```python
from build123d import *

# Parameters (mm, degrees)
F0_R     = 6.35
F1_DEPTH = 31.75
F2_R     = 7.9375
F3_DEPTH = 9.525
F4_DEPTH = 9.525


with BuildPart() as f1:
    # F0 (on Front) → F1 (new body)
    with BuildSketch(Plane.XZ):
        with BuildLine():
            ThreePointArc((-45.625926, 31.75), (-61.553538, 17.067408), (-48.212963, 0))
            Line((-48.212963, 0), (52.916662, 0))
            Line((52.916662, 0), (52.916662, 9.525))
            Line((52.916662, 9.525), (34.337035, 9.525))
            Line((34.337035, 9.525), (34.337035, 22.225))
            Line((34.337035, 22.225), (52.681481, 22.225))
            Line((52.681481, 22.225), (52.681481, 31.75))
            Line((52.681481, 31.75), (-45.625926, 31.75))
        make_face()
        with Locations((-45.625926, 15.769602)):
            Circle(F0_R, mode=Mode.SUBTRACT)
    extrude(amount=-F1_DEPTH)

    # F2 (on Top) → F3 (join, through all)
    with BuildSketch(Plane.XY):
        with BuildLine():
            ThreePointArc((52.916662, 31.75), (37.041662, 15.875), (52.916662, 0))
            ThreePointArc((52.916662, 0), (64.141982, 4.64968), (68.791662, 15.875))
            ThreePointArc((68.791662, 15.875), (64.141982, 27.10032), (52.916662, 31.75))
        make_face()
        with Locations((52.916662, 15.875)):
            Circle(F2_R, mode=Mode.SUBTRACT)
    extrude(amount=F3_DEPTH)

    # F2 (on Top) → F4 (cut, through all)
    with BuildSketch(Plane.XY):
        with Locations((52.916662, 15.875)):
            Circle(F2_R)
    extrude(amount=F4_DEPTH, mode=Mode.SUBTRACT)


solid = f1.part
```
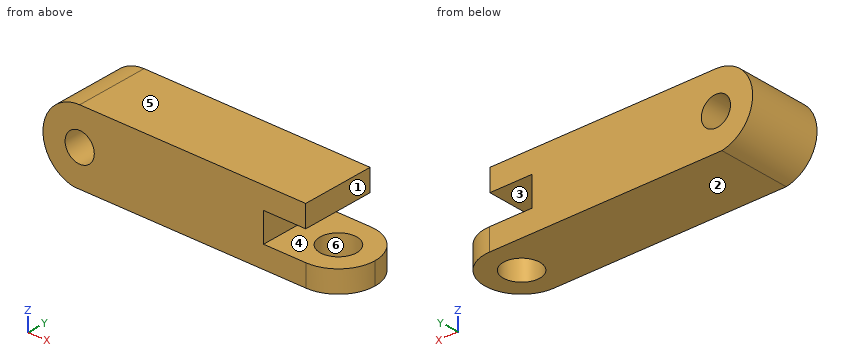
Could you check a few things on this model? Use its own coordinates, in mm. Face numbers are marked on the shaded views. A direction names the side the tool comes from. Round coordinates to 2 decimals unless told otherwise and drop trailing zeros. Loops run counter-clockwise (first coordinate to the right, second up) from the corner with the lowest first, then second, coordinate; pieces in that order, holes last.
Q1. I want a section at B-B (y = 14.5). Write out the boundary of the cut face in (x, z) (3 decimals), and give its area (3 significant figures).
Q2. For P1, Ø5, axis at x = 48.5, z = 11, coming from the +Y side; P2, Ø3, axis at y = 9, z = 26.5, coming from the +X side; P3, Ø5, axis at y = 4, z = 12, coming from the -X side; P4, Ø12, axis at y = 22.5, z = 8, coming from the -X side, each with a flat end and sliding along its axis, tell me the tip position at first contact or that it passes through.
Q3. I want a section at D-D (y = 4). Write out the boundary of the cut face in (x, z) (3 decimals).
Q4. On a 3-axis mill with a long thin cutter (end or side, diameter ignored), from which of +Z, -Z, +X, -X, +Y, -Y can I reach the whole of each face in a straight line? I mean the marked faces 4, 5 and 6. Say none if no direction works.
Q5. Please list where these lines run through material, in increasing order: L1, parallel to X at y = 27, z = 16; L2, parallel to Z at x = 38, y = 21.5 (3 decimals); L3, parallel to X at y = 19, z = 3.5.
Q6. I want a section at C-C (z = 20). Write out the boundary of the cut face in (x, y), and give its area (3 significant figures).
Q7. Thinking about a two-plate mould opening in Z: for the marked faces 1, 2 and 3, which applies, pulls with the +Z half, pulls with the -Z half, needs draft (parallel to the pull), parting line crosses it, or undercut?
Q8. I want a section at A-A (x = 42.5). Write out the boundary of the cut face in (y, z) (3 decimals), and give its area (3 significant figures).
Answer below:
1. outline: (-48.213, 0) - (45.099, 0) - (45.099, 9.525) - (34.337, 9.525) - (34.337, 22.225) - (52.681, 22.225) - (52.681, 31.75) - (-45.626, 31.75) arc R15.98 ccw to start; (60.734, 0) - (68.732, 0) - (68.732, 9.525) - (60.734, 9.525) - close; hole circle Ø12.7 at (-45.626, 15.77)
1. area: 3,170 mm2
2. P1: stops at y = 31.75
2. P2: stops at x = 52.68
2. P3: stops at x = -61.56
2. P4: stops at x = -61.51
3. outline: (-48.213, 0) - (63.452, 0) - (63.452, 9.525) - (34.337, 9.525) - (34.337, 22.225) - (52.681, 22.225) - (52.681, 31.75) - (-45.626, 31.75) arc R15.98 ccw to start; hole circle Ø12.7 at (-45.626, 15.77)
4. face 4: +X, +Y, -Y
4. face 5: +Z, +X, -X, +Y, -Y
4. face 6: -Z
5. L1: x = -61.6 to -51.97, -39.28 to 34.34
5. L2: z = 0 to 9.525, 22.225 to 31.75
5. L3: x = -55.86 to 45.62, 60.21 to 68.48
6. outline: (-61.04, 0) - (-50.36, 0) - (-50.36, 31.75) - (-61.04, 31.75) - close; (-40.89, 0) - (34.34, 0) - (34.34, 31.75) - (-40.89, 31.75) - close
6. area: 2,730 mm2
7. face 1: needs draft
7. face 2: pulls with the -Z half
7. face 3: undercut
8. outline: (0, 0) - (31.75, 0) - (31.75, 9.525) - (0, 9.525) - close; (0, 22.225) - (31.75, 22.225) - (31.75, 31.75) - (0, 31.75) - close
8. area: 605 mm2
